from build123d import *

# Parameters (mm, degrees)
F0_W      = 5.842
F0_H      = 12.7
F0_R      = 3.175
F2_DEPTH  = 3.175
F3_DEPTH  = 6.35
F4_R      = 1.524
F5_DEPTH  = 7.62
F6_DEPTH  = 1.27
F7_R      = 1.524
F8_DEPTH  = 17.78
F9_R      = 1.524
F10_DEPTH = 10.414


with BuildPart() as f1:
    # F0 (on Front) → F1 (revolve)
    with BuildSketch(Plane.XZ):
        Polygon((5.842, 12.7), (5.842, 0), (66.294, 0), (66.294, 12.7), (56.134, 12.7), (56.134, 10.16), (10.16, 10.16), (10.16, 12.7), align=None)
    revolve(axis=Axis((-3.3274, 0, 0), (-1, 0, 0)))

    # F0 (on Front) → F2 (join, symmetric)
    with BuildSketch(Plane.XZ):
        with BuildLine():
            Line((-0.9398, 0), (0, 0))
            Line((0, 0), (0, 12.7))
            Line((0, 12.7), (5.842, 12.7))
            Line((5.842, 12.7), (5.842, 15.24))
            Line((5.842, 15.24), (-0.508, 15.24))
            Line((-0.508, 15.24), (-10.8806298187, 3.8475430269))
            ThreePointArc((-10.8806298187, 3.8475430269), (-4.5919612295, 5.3297205562), (-0.9398, 0))
        make_face()
        with BuildLine():
            Line((5.842, 0), (0, 0))
            Line((0, 0), (-0.9398, 0))
            ThreePointArc((-0.9398, 0), (-3.1957909266, -4.5493385486), (-8.1826630726, -5.5069827884))
            Line((-8.1826630726, -5.5069827884), (5.842, -9.398))
            Line((5.842, -9.398), (5.842, 0))
        make_face()
        with Locations((2.921, 6.35)):
            Rectangle(F0_W, F0_H)
        with BuildLine():
            ThreePointArc((-8.1826630726, -5.5069827884), (-3.1957909266, -4.5493385486), (-0.9398, 0))
            ThreePointArc((-0.9398, 0), (-4.5919612295, 5.3297205562), (-10.8806298187, 3.8475430269))
            ThreePointArc((-10.8806298187, 3.8475430269), (-12.1459778134, -1.5837270034), (-8.1826630726, -5.5069827884))
        make_face()
        with Locations((-6.6548, 0)):
            Circle(F0_R, mode=Mode.SUBTRACT)
    extrude(amount=F2_DEPTH, both=True)

    # F3 (add): a face of the model
    f3_faces = [f1.faces().sort_by_distance(p)[0] for p in [
        (5.842, 3.5313700488, 1.4493610621),
    ]]
    extrude(f3_faces, amount=F3_DEPTH)

    # F4 (on face) → F5 (join)
    with BuildSketch(Plane.YZ.offset(66.294)):
        with BuildLine():
            ThreePointArc((-5.08, 0), (0, 5.08), (5.08, 0))
            Line((5.08, 0), (5.08, 11.6397422652))
            ThreePointArc((5.08, 11.6397422652), (0, 12.7), (-5.08, 11.6397422652))
            Line((-5.08, 11.6397422652), (-5.08, 0))
        make_face()
        with BuildLine():
            ThreePointArc((-5.08, 0), (0, -5.08), (5.08, 0))
            ThreePointArc((5.08, 0), (0, 5.08), (-5.08, 0))
        make_face()
        Circle(F4_R, mode=Mode.SUBTRACT)
        with BuildLine():
            ThreePointArc((-5.08, 11.6397422652), (0, 12.7), (5.08, 11.6397422652))
            Line((5.08, 11.6397422652), (5.08, 15.24))
            Line((5.08, 15.24), (-5.08, 15.24))
            Line((-5.08, 15.24), (-5.08, 11.6397422652))
        make_face()
    extrude(amount=F5_DEPTH)

    # F6 (add): a face of the model
    f6_faces = [f1.faces().sort_by_distance(p)[0] for p in [
        (66.294, 0, 13.7792682875),
    ]]
    extrude(f6_faces, amount=F6_DEPTH)

    # F7 (on face) → F8 (cut)
    with BuildSketch(Plane.XY.offset(15.24)):
        with Locations((2.667, 0)):
            Circle(F7_R)
    extrude(amount=-F8_DEPTH, mode=Mode.SUBTRACT)

    # F9 (on face) → F10 (cut)
    with BuildSketch(Plane.XY.offset(15.24)):
        with Locations((69.469, 0)):
            Circle(F9_R)
    extrude(amount=-F10_DEPTH, mode=Mode.SUBTRACT)


solid = f1.part
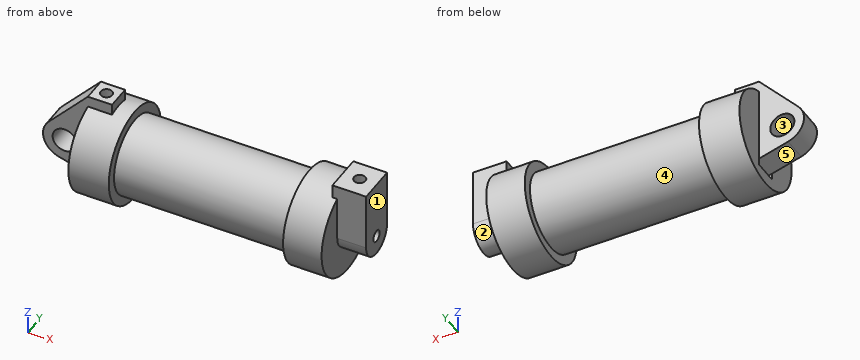
Read the model definition and answer for the solid it produces. Units are mm, in the model's axes. Face numbers are marked on the shaded views. A direction names the side the tool comes from. Give positions to 0.01 mm unless a question says otherwise; leave off trailing zeros. Write each loop counter-clockwise with the first axis right and the second up, starting at its lowest first coordinate (ties: lowest second). Pieces come first, ordered by that corner, then holes. Notation, with made-up numbers: M 60,67 L 117,67 A16 ccw 117,72 Z; hole C -16.75,1.5 d1. An arc over 180 degrees is marked long. One line per item, written item: value. Start each with the question number.
(1) Find section B-B (y = 7.25). Determine the outline of the cut face in (x, z).
(2) Find section A-A (z = 7.5). Determine the outline of the cut face in (x, y) (3 decimals), plus the area to 3 significant figures.
(3) Determine the mould class of the marked faces 3, 4 and 5 for opening direction Y: pulls with the +Y half, pulls with the -Y half, needs draft (parallel to the pull), parting line crosses it, or undercut.
(4) Flat-ended cylindrical pins translate along their axes: pin 1 Ø12 at (x, z) = (36.5, -9) entering from +Y; pin 2 Ø4 at (x, y) = (69.469, 0) entering from -Z; pin 3 Ø6 at (x, z) = (-0.5, -3.5) entering from -Y. Find the tip coordinate at first contact, or state that the pin passes through.
(5) Find the intervals of material crossed by line 1 (Z direction, x = 70.25, y = 0); line 2 (Y direction, x = 31, z = 0); line 3 (X direction, y = -4, z = 9), in increasing order.
(6) Find section D-D (y = -8.25). Determine the outline of the cut face in (x, z), plus the area to 3 significant figures.
(7) Find section C-C (x = 29.5). Determine the outline of the cut face in (y, z).
(8) A tool of negligible diameter and unlimited length cuts with its end or side. For the marked faces 1 and 2, from which of +Z, -Z, +X, -X, +Y, -Y can it reach the whole face along a straight path? Write none if from no direction.
Results below:
1. outline: M -0.51,-10.43 L 10.16,-10.43 L 10.16,-7.12 L 56.13,-7.12 L 56.13,-10.43 L 66.29,-10.43 L 66.29,10.43 L 56.13,10.43 L 56.13,7.12 L 10.16,7.12 L 10.16,10.43 L -0.51,10.43 Z
2. outline: M -7.555,-3.175 L -0.508,-3.175 L -0.508,-10.249 L 10.16,-10.249 L 10.16,-6.854 L 56.134,-6.854 L 56.134,-10.249 L 66.294,-10.249 L 66.294,-5.08 L 73.914,-5.08 L 73.914,5.08 L 66.294,5.08 L 66.294,10.249 L 56.134,10.249 L 56.134,6.854 L 10.16,6.854 L 10.16,10.249 L -0.508,10.249 L -0.508,3.175 L -7.555,3.175 Z; hole C 2.667,0 d3.048; hole C 69.469,0 d3.048
2. area: 1,160 mm^2
3. face 3: needs draft
3. face 4: parting line crosses it
3. face 5: undercut
4. pin 1: stops at y = 9.71
4. pin 2: stops at z = -5.08
4. pin 3: stops at y = -12.69
5. line 1: z = -5.08 to -1.52, 1.52 to 4.83
5. line 2: y = -10.16 to 10.16
5. line 3: x = -0.51 to 73.91
6. outline: M -0.51,-9.66 L 10.16,-9.66 L 10.16,-5.93 L 56.13,-5.93 L 56.13,-9.66 L 66.29,-9.66 L 66.29,9.66 L 56.13,9.66 L 56.13,5.93 L 10.16,5.93 L 10.16,9.66 L -0.51,9.66 Z
6. area: 947 mm^2
7. outline: C 0,0 d20.32
8. face 1: +Z, -Z, +X, +Y, -Y
8. face 2: -Z, +X
